Verification items for the finished model (mm, model axes). Face numbers are marked on the shaded views. A direction names the side the tool comes from. Give positions to 0.01 mm unless a question says otherwise; leave off trailing zeros. Loops run counter-clockwise (first coordinate to the right, second up) from the corner with the lowest first, then second, coordinate; pieces in that order, holes last. Notation, with made-up numbers: (54.5, 34) -> (71.5, 34) arc R20 ccw to (71.5, 67) -> close; hole circle Ø10 at (55.5, -16). An arc over 180 degrees is marked (long way). Answer in a Markdown table with one row per item. Add a question column.
Q1. Section check A-A on x = 3.5. Enter the section's corners in (y, z), and give its area (3 significant figures).
Q2. Gauge pin test, flat ends, axial feed: P1, Ø2, axis at x = -5, z = 27, coming from the +Y side; P2, Ø1, axis at x = -8.5, z = 157.5, coming from the +Y side; P3, Ø8, axis at y = -6, z = 67.5, coming from the +X side. Record the tip position at first contact, or that the pin passes through.
Q3. Set-up check for the marked faces 1 and 2: record each of +Z, -Z, +X, -X, +Y, -Y from which the full face is reachable in a straight line by a thin tool's end or side.
Q4. Material ranges on probe 1 along Y at (x, z) = (0, 65) (3 decimals); probe 2 along X at (y, z) = (8.5, 180.5); probe 3 along X at (y, z) = (-8, 43), recorded low to high.
Q5. Section check B-B on z = 104.5. Enter the section's corners in (x, y) (3 decimals), and give its area (3 significant figures).
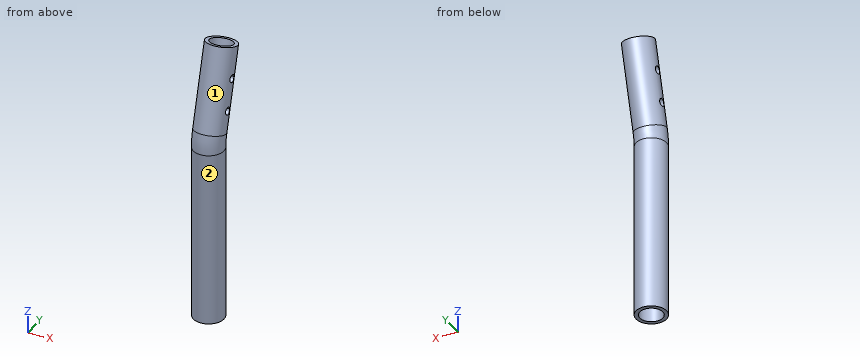
```python
from build123d import *

# Parameters (mm, degrees)
F0_R     = 12.7
F0_R_2   = 9.525
F3_DEPTH = 25.4


with BuildPart() as f2:
    # F2: sweep along a path in F1
    with BuildLine(Plane.YZ) as f2_path:
        Line((0, 0), (0, 145.7120531226))
        ThreePointArc((0, 145.7120531226), (0.4346010422, 152.3427836873), (1.7309680245, 158.8600606138))
        Line((1.7309680245, 158.8600606138), (19.7220112368, 226.0035479632))
    # F0 (on Top) → F2 (sweep)
    with BuildSketch(Plane.XY):
        Circle(F0_R)
        Circle(F0_R_2, mode=Mode.SUBTRACT)
    sweep(path=f2_path.line)

    # F1 (on Right) → F3 (cut, symmetric)
    with BuildSketch(Plane.YZ):
        with BuildLine():
            ThreePointArc((13.9697579594, 204.535846474), (10.0811929927, 202.2907824437), (12.326257023, 198.402217477))
            Line((12.326257023, 198.402217477), (13.9697579594, 204.535846474))
        make_face()
        with BuildLine():
            Line((13.9697579594, 204.535846474), (12.326257023, 198.402217477))
            ThreePointArc((12.326257023, 198.402217477), (15.0808250283, 198.9501351201), (16.3230074912, 201.4690319755))
            ThreePointArc((16.3230074912, 201.4690319755), (15.6669043466, 203.4018495126), (13.9697579594, 204.535846474))
        make_face()
        with BuildLine():
            Line((7.3957542138, 180.0013304862), (5.7522532774, 173.8677014893))
            ThreePointArc((5.7522532774, 173.8677014893), (8.5068212827, 174.4156191323), (9.7490037456, 176.9345159877))
            ThreePointArc((9.7490037456, 176.9345159877), (9.092900601, 178.8673335248), (7.3957542138, 180.0013304862))
        make_face()
        with BuildLine():
            ThreePointArc((7.3957542138, 180.0013304862), (3.5071892471, 177.7562664559), (5.7522532774, 173.8677014893))
            Line((5.7522532774, 173.8677014893), (7.3957542138, 180.0013304862))
        make_face()
    extrude(amount=F3_DEPTH, both=True, mode=Mode.SUBTRACT)


solid = f2.part
```
Taken from the geometry:
| question | item | result |
|---|---|---|
| 1 | outline | (-12.21, 0) -> (-8.86, 0) -> (-8.86, 145.71) arc R59.66 cw to (-6.83, 161.15) -> (11.17, 228.3) -> (7.93, 229.16) -> (-10.06, 162.02) arc R63.01 ccw to (-12.21, 145.71) -> close; (8.86, 0) -> (12.21, 0) -> (12.21, 145.71) arc R38.59 cw to (13.52, 155.7) -> (31.51, 222.84) -> (28.28, 223.71) -> (10.29, 156.57) arc R41.94 ccw to (8.86, 145.71) -> close |
| 1 | area | 1,530 mm² |
| 2 | P1 | stops at y = 12.05 |
| 2 | P2 | stops at y = 11.6 |
| 2 | P3 | stops at x = 12.54 |
| 3 | face 1 | none |
| 3 | face 2 | -Z |
| 4 | probe 1 | y = -12.7 to -9.525, 9.525 to 12.7 |
| 4 | probe 2 | x = -12.67 to -9.48, 9.48 to 12.67 |
| 4 | probe 3 | x = -9.86 to -5.17, 5.17 to 9.86 |
| 5 | outline | circle Ø25.4 at (0, 0); hole circle Ø19.05 at (0, 0) |
| 5 | area | 222 mm² |
